Check sheet for the modelled part. Datum: model origin and axes. Units: mm. A direction names the side the tool comes from. Round coordinates to 2 decimals unless told otherwise and drop trailing zeros. Write each loop counter-clockwise with the first axis right and the second up, starting at its lowest first coordinate (ties: lowest second). Pieces come first, ordered by that corner, then holes. Notation, with made-up numbers: M -32.5,46.25 L 4.5,46.25 A7 ccw 4.5,58.25 Z; hole C -11.5,-20.75 d7. An arc over 180 degrees is marked long. One line per item, written item: value.
Autodesk Inventor part; units mm, degrees
ref_plane "YZ Plane" through (0, 0, 0) normal (1, 0, 0) x (0, 1, 0)
ref_plane "XZ Plane" through (0, 0, 0) normal (0, 1, 0) x (-1, 0, 0)
ref_plane "XY Plane" through (0, 0, 0) normal (0, 0, 1) x (1, 0, 0)
sketch "Sketch1" plane through (0, 0, 0) normal (0, 0, 1) x (1, 0, 0)
  line L0 (-12.1708, 16.0073) -> (13.2292, 16.0073)
  line L1 (13.2292, 16.0073) -> (13.2292, -34.7927)
  line L2 (13.2292, -34.7927) -> (-12.1708, -34.7927)
  line L3 (-12.1708, -34.7927) -> (-12.1708, 16.0073)
  line L4 (11.9592, 14.7373) -> (-10.9008, 14.7373)
  line L5 (-10.9008, 14.7373) -> (-10.9008, -33.5227)
  line L6 (-10.9008, -33.5227) -> (11.9592, -33.5227)
  line L7 (11.9592, -33.5227) -> (11.9592, 14.7373)
  point P0 (0, 0)
  dimension "d0" = 25.4
  dimension "d1" = 50.8
  dimension "d2" = 1.27
extrude "Extrusion1" add sketch "Sketch1" along normal blind 76.2
sketch "Sketch2" plane through (-12.1708, 16.0073, 0) normal (0, 1, 0) x (1, 0, 0)
  circle A0 centre (12.7, -12.7) radius 1.7272
  line L0 (25.4, 0) -> (0, 0)
  line L1 (0, 0) -> (0, -76.2)
  point P0 (12.1708, 0)
  dimension "d5" = 3.4544
  dimension "d6" = 12.7
  dimension "d7" = 12.7
extrude "Extrusion2" cut sketch "Sketch2" against normal through all
pattern_linear "Rectangular Pattern1" count 8 spacing 25.4 along (0, 0, 1) of "Extrusion2"
sketch "Sketch3" plane through (13.2292, -34.7927, 0) normal (1, 0, 0) x (0, 0, -1)
  circle A0 centre (-44.45, 25.4) radius 14.2875
  line L0 (0, 0) -> (0, 50.8)
  line L1 (-76.2, 0) -> (-76.2, 50.8)
  circle A1 centre (-69.85, 25.4) radius 2.5781
  circle A2 centre (-19.05, 25.4) radius 2.5781
  line L2 (-76.2, 50.8) -> (-76.2, 0) construction
  line L3 (-76.2, 25.4) -> (0, 25.4) construction
  line L4 (0, 1.27) -> (0, 49.53) construction
  line L5 (0, 0) -> (-76.2, 0) construction
  point P0 (0, 34.7927)
  dimension "d15" = 28.575
  dimension "d19" = 31.75
  dimension "d20" = 5.1562
  dimension "d21" = 5.1562
  dimension "d22" = 25.4
  dimension "d23" = 25.4
  dimension "d24" = 25.4
extrude "Extrusion3" cut sketch "Sketch3" against normal through all contours A0
extrude "Extrusion4" cut sketch "Sketch3" against normal through all contours A1 | A2
equation "\"d3\" = d13"
equation "\"d10\" = d14"
equation "\"d13\" = 76.2"
equation "\"d14\" = d13"
properties part number "VerseFrame 5in STOCK"
Q1. Draft check along X on faces 1 (the cylindrical face through (0.3, 15.38, 10.99)), 2 (the flat face through (-12.171, -10, 29)), 3 (the flat face through (13.229, -9, 29)), 4 (the cylindrical face through (12.603, -10.961, 21.096)). Enter one of: pulls with the +X half, pulls with the -X half, needs draft (parallel to the pull), parting line crosses it, or undercut.
Completed:
face 1: undercut
face 2: pulls with the -X half
face 3: pulls with the +X half
face 4: needs draft
Q2. Scan lines: line 1 (X direction, y = 4.5, z = 65); line 2 (Y direction, x = -3, z = 48.5); line 3 (Y direction, x = -11.65, z = 44.45). Record each from-to range of solid material in increasing order. Write a range as [from, to].
Completed:
line 1: [-12.17, -10.9], [11.96, 13.23]
line 2: [-34.79, -33.52], [14.74, 16.01]
line 3: [-34.79, -23.68], [4.89, 16.01]
Q3. Access from +Z, -Z, +X, -X, +Y, -Y to the whole of each face (thin tool, end or side, straight path). Record for faces 5 (the cylindrical face through (-11.527, -10.961, 21.096)), 6 (the flat face through (-2, 14.737, 38)).
Completed:
face 5: +X, -X
face 6: +Z, -Z
Q4. Sectioned sample at C-C on x = -2. Enter the section's corners in (y, z), and give its area (3 significant figures).
Completed:
outline: M -34.79,0 L -33.52,0 L -33.52,76.2 L -34.79,76.2 Z; M 14.74,0 L 16.01,0 L 16.01,76.2 L 14.74,76.2 Z
area: 194 mm^2
Q5. Depth check by flat-ended pin: P1, Ø4, axis at x = 0.53, z = 12.7, coming from the +Y side. Enter the tip coordinate at first touch or a pass-through.
Completed:
P1: y = 16.01
Q6. Sectioned sample at B-B on y = -31. Enter the section's corners in (x, z), and give its area (3 significant figures).
Completed:
outline: M -12.17,0 L -10.9,0 L -10.9,76.2 L -12.17,76.2 Z; M 11.96,0 L 13.23,0 L 13.23,76.2 L 11.96,76.2 Z
area: 194 mm^2
Q7. Sectioned sample at D-D on z = 38.1. Enter the section's corners in (x, y), and give its area (3 significant figures).
Completed:
outline: M -12.17,-34.79 L -1.2,-34.79 L -1.2,-33.52 L -10.9,-33.52 L -10.9,-22.19 L -12.17,-22.19 Z; M -12.17,3.41 L -10.9,3.41 L -10.9,14.74 L -1.2,14.74 L -1.2,16.01 L -12.17,16.01 Z; M 2.26,-34.79 L 13.23,-34.79 L 13.23,-22.19 L 11.96,-22.19 L 11.96,-33.52 L 2.26,-33.52 Z; M 2.26,14.74 L 11.96,14.74 L 11.96,3.41 L 13.23,3.41 L 13.23,16.01 L 2.26,16.01 Z
area: 113 mm^2
Q8. Sectioned sample at A-A on z = 63.5. Enter the section's corners in (x, y), and give its area (3 significant figures).
Completed:
outline: M -12.17,-34.79 L -1.2,-34.79 L -1.2,-33.52 L -10.9,-33.52 L -10.9,14.74 L -1.2,14.74 L -1.2,16.01 L -12.17,16.01 Z; M 2.26,-34.79 L 13.23,-34.79 L 13.23,16.01 L 2.26,16.01 L 2.26,14.74 L 11.96,14.74 L 11.96,-33.52 L 2.26,-33.52 Z
area: 178 mm^2
